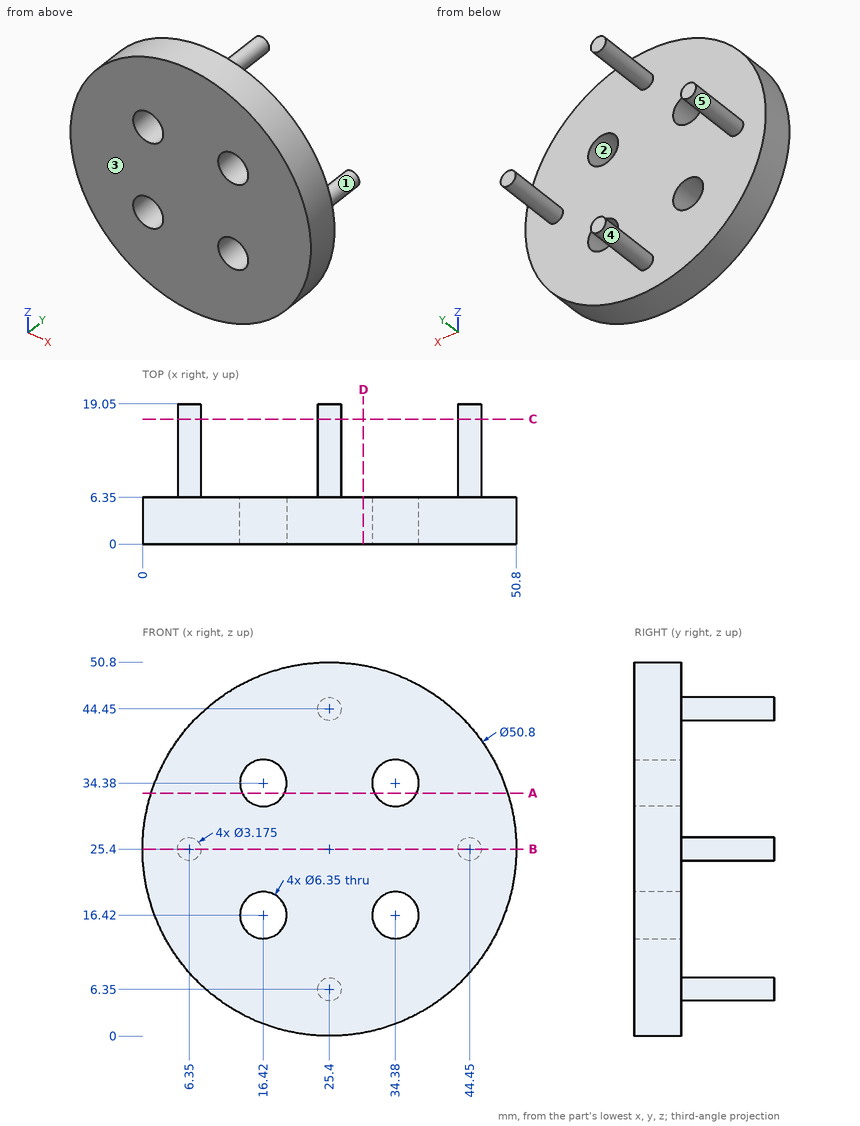
Could you check a few things on this drawing? It's one solid part, dimensions in mm from its lowest x, y, z. A direction names the side the tool comes from. Coordinates: 2 decimals unless noted, no trailing zeros. Loops run counter-clockwise (first coordinate to the right, second up) from the corner with the lowest first, then second, coordinate; pieces in that order, holes last.
1. Imagine slicing it at A-A (z = 33). Please give me the cut outline in (x, y).
2. Imagine slicing it at C-C (y = 17). Give the number of separate pieces and of enclosed holes in the cut face.
3. Imagine slicing it at D-D (x = 30). Please give me the cut outline in (y, z).
4. For P1, Ø7.5, axis at x = 34.38, z = 16.42, coming from the +Y side; P2, Ø10, axis at y = 2, z = 11.5, coming from the -X side; P3, Ø5, axis at x = 29, y = 5, coming from the -Z side, each with a flat end and sliding along its axis, tell me the tip position at first contact or that it passes through.
5. We'd pull the mould along X, two halves only. Please class the marked faces 3, 4 and 5: released by +X, released by -X, zero draft, split by the parting line, or undercut.
6. I need wall thicknesses on L1, parallel to X at y = 2, z = 15.5; L2, parallel to Z at x = 34, y = 4; L3, parallel to Y at x = 32, z = 14. Which ranges of each line are inside material? Lowest first, please.
7. For the marked faces 1 and 2, which set-ups out of +Z, -Z, +X, -X, +Y, -Y let a thin tool reach every point of the face, with its end or its side?
8. Imagine slicing it at B-B (z = 25.4). Please give me the cut outline in (x, y).
Computed values:
1. outline: (1.16, 0) - (13.56, 0) - (13.56, 6.35) - (1.16, 6.35) - close; (19.28, 0) - (31.52, 0) - (31.52, 6.35) - (19.28, 6.35) - close; (37.24, 0) - (49.64, 0) - (49.64, 6.35) - (37.24, 6.35) - close
2. separate pieces: 4
2. enclosed holes: 0
3. outline: (0, 0.42) - (6.35, 0.42) - (6.35, 50.38) - (0, 50.38) - close
4. P1: stops at y = 6.35
4. P2: stops at x = 1.61
4. P3: stops at z = 0.02
5. face 3: zero draft
5. face 4: split by the parting line
5. face 5: undercut
6. L1: x = 2.01 to 13.38, 19.46 to 31.34, 37.42 to 48.79
6. L2: z = 1.5 to 13.27, 19.57 to 31.23, 37.53 to 49.3
6. L3: y = 0 to 6.35
7. face 1: +Y
7. face 2: +Y, -Y
8. outline: (0, 0) - (50.8, 0) - (50.8, 6.35) - (46.04, 6.35) - (46.04, 19.05) - (42.86, 19.05) - (42.86, 6.35) - (7.94, 6.35) - (7.94, 19.05) - (4.76, 19.05) - (4.76, 6.35) - (0, 6.35) - close
